For this review, use the dimensioned drawing (mm, ordinates from the lowest corner) and the shaded views. A direction names the side the tool comes from. Coordinates: 2 decimals unless noted, no trailing zeros. Order: outer loops, then holes, each group sorted by start corner. A loop starts at its lowest first (then second) coordinate and runs counter-clockwise, first axis right, second up. Notation, with made-up numbers: M 60.25,6 L 83.25,6 A22 cw 83.25,30 Z; hole C 6,-35.5 d8. An arc over 180 degrees is marked long. Use one line per item in the form item = value. Start each with the question number.
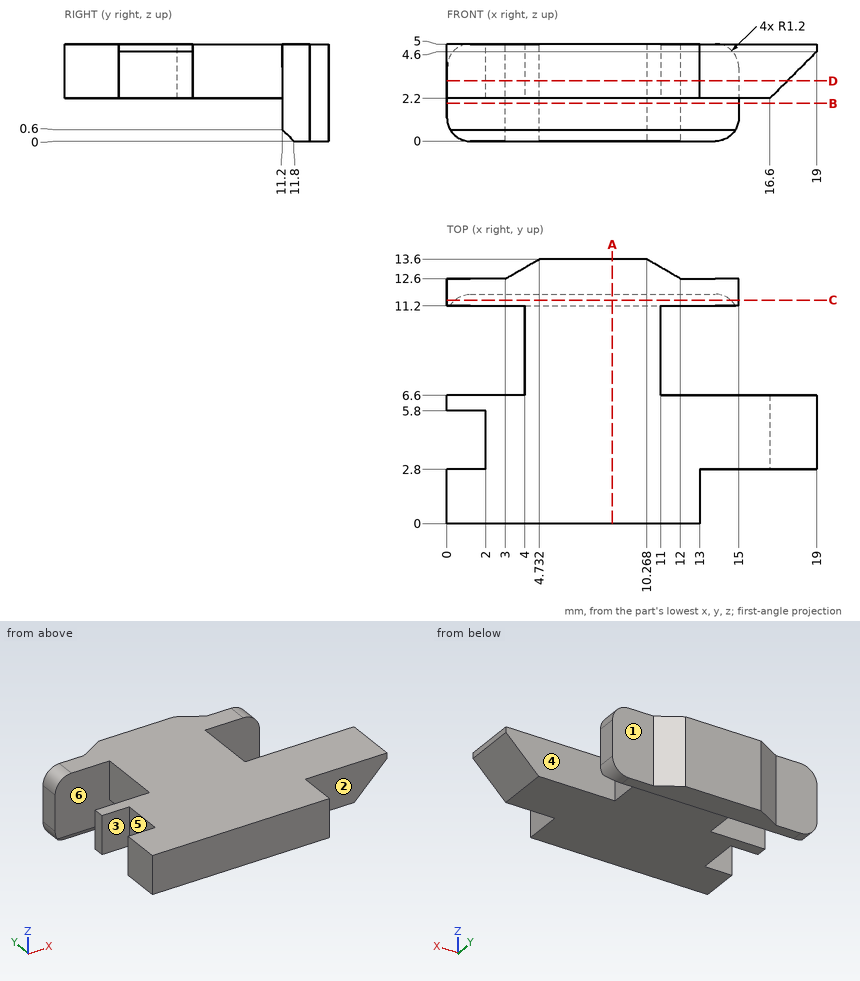
1. Consider section B-B, the plane z = 1.95. Write out the cut boundary in (x, y).
2. Consider section D-D, the plane z = 3.1. Write out the cut boundary in (x, y).
3. For pin 1 Ø3.5 at (x, y) = (10.5, 6) entering from -Z; pin 2 Ø1.4 at (y, z) = (4, 4.5) entering from -X; pin 3 Ø1.5 at (x, z) = (13.5, 2) entering from +Y, all flat-tipped, find the tip position at first contact; note any pin that passes through.
4. To check wall thickness, follow line 1 (Y direction, x = 12.25, z = 4.35); line 2 (X direction, y = 2.25, z = 3.65); line 3 (Z direction, x = 9.25, y = 2.5). State the ranges of each line that lie inside material, in increasing order.
5. Consider section C-C, the plane y = 11.5. Write out the cut boundary in (x, z).
6. Consider section A-A, the plane x = 8.5. Write out the cut boundary in (y, z).
7. Tool access review of the marked faces 4, 5 and 6: name each direction out of +Z, -Z, +X, -X, +Y, -Y from which nothing blocks a thin tool from reaching the whole face with its end or side.
8. The part is to be moulded in two halves that separate along Y. For the marked faces 1, 2 and 3, say which applies: pulls with the +Y half, pulls with the -Y half, needs draft (parallel to the pull), parting line crosses it, or undercut.
Answers follow:
q1.outline = M 0,11.2 L 15,11.2 L 15,12.6 L 12,12.6 L 10.27,13.6 L 4.73,13.6 L 3,12.6 L 0,12.6 Z
q2.outline = M 0,0 L 13,0 L 13,2.8 L 17.5,2.8 L 17.5,6.6 L 11,6.6 L 11,11.2 L 15,11.2 L 15,12.6 L 12,12.6 L 10.27,13.6 L 4.73,13.6 L 3,12.6 L 0,12.6 L 0,11.2 L 4,11.2 L 4,6.6 L 0,6.6 L 0,5.8 L 2,5.8 L 2,2.8 L 0,2.8 Z
q3.pin_1 = 2.2
q3.pin_2 = 2
q3.pin_3 = 12.6
q4.line_1 = 0 to 6.6, 11.2 to 12.6
q4.line_2 = 0 to 13
q4.line_3 = 2.2 to 5
q5.outline = M 0,1.2 A1.2 ccw 0.41,0.3 L 14.59,0.3 A1.2 ccw 15,1.2 L 15,3.8 A1.2 ccw 13.8,5 L 1.2,5 A1.2 ccw 0,3.8 Z
q6.outline = M 0,2.2 L 11.2,2.2 L 11.2,0.6 L 11.8,0 L 13.6,0 L 13.6,5 L 0,5 Z
q7.face_4 = +Z, -Z, +X
q7.face_5 = +Z, -Z, -X
q7.face_6 = -Z
q8.face_1 = pulls with the +Y half
q8.face_2 = pulls with the -Y half
q8.face_3 = undercut
